CAD build for the part. Positions are in the model's coordinates, mm. A direction names the side the tool comes from. Give positions to 0.01 mm unless a question says otherwise; leave off trailing zeros. Order: outer loops, then holes, each group sorted by start corner. A loop starts at its lowest first (then second) coordinate and runs counter-clockwise, first axis right, second up.
Item 1: Two-plate mould, pull along Y, no slides. Class faces 1 (the flat face through (-39, 1, -10)), 2 (the cylindrical face through (-1.014, 5.824, -8.646)), 3 (the flat face through (-38, 2, -6)): released by +Y, released by -Y, zero draft, split by the parting line, or undercut.
Item 2: Band-saw the part on A-A on y = 6.5. Give the cut face in (x, z), plus the area to 3 significant figures.
Item 3: Which spindle directions (+Z, -Z, +X, -X, +Y, -Y) get a long thin tool onto all of the face, cutting with end or side? Do faces 4 (the flat face through (-77, 4, -5)), 5 (the flat face through (-2, 6, -4)). Say none if no direction does.
Item 4: Band-saw the part on B-B on z = -6.5. Give the cut face in (x, y).
Item 5: Wall check: L1, parallel to X at y = 7.5, z = -2.25; L2, parallel to Y at x = -76.1, z = -6.5; L3, parallel to Z at x = -75.4, y = 6.5. Give the ranges that are in metal, low to high.
Item 6: Band-saw the part on C-C on x = -64.5. Give the cut face in (y, z), plus the area to 3 significant figures.
Item 7: Flat gauge pins, fed straight in: P1, Ø3, axis at y = 2, z = -2, coming from the +X side; P2, Ø3, axis at x = -63.5, y = 5, coming from the -Z side; P3, Ø2, axis at x = -22.5, z = -7, coming from the +Y side. Where does each tip first touch, or does it go through?
Autodesk Inventor part; units mm, degrees
ref_plane "YZ Plane" through (0, 0, 0) normal (1, 0, 0) x (0, 1, 0)
ref_plane "XZ Plane" through (0, 0, 0) normal (0, 1, 0) x (-1, 0, 0)
ref_plane "XY Plane" through (0, 0, 0) normal (0, 0, 1) x (1, 0, 0)
sketch "Sketch1" plane through (0, 0, 0) normal (0, 1, 0) x (-1, 0, 0)
  line L0 (0, 0) -> (77, 0)
  line L1 (77, 0) -> (77, -10)
  line L2 (77, -10) -> (0, -10)
  line L3 (0, -10) -> (0, 0)
  line L4 (77, 0) -> (0, 0)
  line L5 (0, 0) -> (0, -2)
  line L6 (0, -2) -> (77, -2)
  line L7 (77, -2) -> (77, 0)
  point P0 (77, -2)
  point P1 (77, -5)
  dimension "d1" = 10
  dimension "d3" = 2
  dimension "d19" = 77
extrude "Extrusion1" add sketch "Sketch1" along normal blind 2 contours L6 L1 L2 L3
extrude "Extrusion2" add sketch "Sketch1" along normal blind 10 contours L0 L1 L6 L3
sketch "Sketch2" plane through (0, 0, -10) normal (1, 0, 0) x (0, 0, -1)
  line L0 (-10, 0) -> (0, 0)
  line L1 (-10, 0) -> (0, 0)
  line L2 (0, 0) -> (0, 10)
  line L3 (0, 10) -> (-10, 10)
  line L4 (-10, 10) -> (-10, 0)
  dimension "d8" = 10
  dimension "d9" = 10
extrude "Extrusion3" add sketch "Sketch2" against normal blind 2
sketch "Sketch3" plane through (-77, 0, -10) normal (-1, 0, 0) x (0, 0, 1)
  line L0 (0, 0) -> (0, 10)
  line L1 (10, 10) -> (0, 10)
  line L2 (0, 0) -> (10, 0)
  line L3 (10, 0) -> (10, 10)
  line L4 (10, 10) -> (0, 10)
  line L5 (0, 10) -> (0, 0)
  point P0 (10, 0)
extrude "Extrusion4" add sketch "Sketch3" against normal blind 2
sketch "Sketch5" plane through (0, 0, 0) normal (1, 0, 0) x (0, 0, -1)
  line L0 (0, 10) -> (10, 10)
  line L1 (10, 0) -> (10, 10)
  point P0 (0, 0)
  point P1 (6.5, 6.5)
  dimension "d23" = 3.5
  dimension "d24" = 3.5
hole "Hole1" at (0, 6.5, -6.5) direction (-1, 0, 0) diameter 4.5 end through all
properties part number "Legs"
The answers:
1. face 1: zero draft
1. face 2: undercut
1. face 3: released by +Y
2. outline: (-77, -10) - (-75, -10) - (-75, -8.75) - (-77, -8.75) - close; (-77, -4.25) - (-75, -4.25) - (-75, -2) - (-2, -2) - (-2, -4.25) - (0, -4.25) - (0, 0) - (-77, 0) - close; (-2, -10) - (0, -10) - (0, -8.75) - (-2, -8.75) - close
2. area: 168 mm2
3. face 4: +Z, -Z, -X, +Y, -Y
3. face 5: -Z, +Y
4. outline: (-77, 0) - (0, 0) - (0, 4.25) - (-2, 4.25) - (-2, 2) - (-75, 2) - (-75, 4.25) - (-77, 4.25) - close; (-77, 8.75) - (-75, 8.75) - (-75, 10) - (-77, 10) - close; (-2, 8.75) - (0, 8.75) - (0, 10) - (-2, 10) - close
5. L1: x = -77 to -75, -2 to 0
5. L2: y = 0 to 4.25, 8.75 to 10
5. L3: z = -10 to -8.75, -4.25 to 0
6. outline: (0, -10) - (2, -10) - (2, -2) - (10, -2) - (10, 0) - (0, 0) - close
6. area: 36.0 mm2
7. P1: stops at x = 0
7. P2: stops at z = -2
7. P3: stops at y = 2
